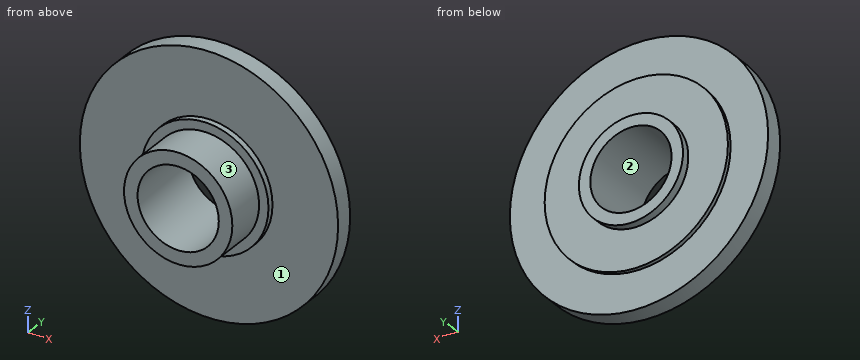
from build123d import *

# Parameters (mm, degrees)
SKETCH3_R          = 19.5
CUT_EXTRUDE1_DEPTH = 50


with BuildPart() as part:
    # Sketch2 → Revolve1 (revolve)
    with BuildSketch(Plane.XY):
        Polygon((0, 0), (26, 0), (26, 20), (30.5, 20), (30.5, 23), (62, 23), (62, 32), (44, 32), (44, 34), (25, 34), (25, 38), (0, 38), align=None)
    revolve(axis=Axis((0, 0, 0), (0, 1, 0)))

    # Sketch3 → Cut-Extrude1 (cut)
    with BuildSketch(Plane(origin=(0, 38, 0), x_dir=(1, 0, 0), z_dir=(0, 1, 0))):
        Circle(SKETCH3_R)
    extrude(amount=-CUT_EXTRUDE1_DEPTH, mode=Mode.SUBTRACT)


solid = part.part
Work out the finished part from the listing and answer in its coordinate system (mm). Face numbers are marked on the shaded views. Give positions to 0.01 mm unless a question says otherwise; leave off trailing zeros. Loops run counter-clockwise (first coordinate to the right, second up) from the corner with the lowest first, then second, coordinate; pieces in that order, holes last. Notation, with made-up numbers: M 36.5,4 L 62.5,4 A31 ccw 62.5,30 Z; hole C -5,44 d3. An arc over 180 degrees is marked long. Use CSV: the item, a comma, the result in double quotes.
1) Consider L1, parallel to Z at x = 0, y = 27; L2, parallel to Y at x = 16.5, z = -39. Determine where each line is inside the solid, lowest interval first.
Answer:
L1,"-62 to -19.5, 19.5 to 62"
L2,"23 to 34"
2) Find section B-B on z = 0. Write down the section's boundary in (x, y), plus the area to 3 significant figures.
Answer:
outline,"M -62,23 L -30.5,23 L -30.5,20 L -26,20 L -26,0 L -19.5,0 L -19.5,38 L -25,38 L -25,34 L -44,34 L -44,32 L -62,32 Z; M 19.5,0 L 26,0 L 26,20 L 30.5,20 L 30.5,23 L 62,23 L 62,32 L 44,32 L 44,34 L 25,34 L 25,38 L 19.5,38 Z"
area,"1,230 mm^2"
3) Determine the mould class of the marked faces 1, 2 and 3 for opening direction X: released by +X, released by -X, zero draft, split by the parting line, or undercut.
Answer:
face 1,"zero draft"
face 2,"undercut"
face 3,"split by the parting line"
4) Find section C-C on x = 34. Write down the section's boundary in (y, z).
Answer:
outline,"M 23,-51.85 L 32,-51.85 L 32,-27.93 L 34,-27.93 L 34,27.93 L 32,27.93 L 32,51.85 L 23,51.85 Z"
5) Given P1, Ø4, axis at x = -5.5, y = 19, coming from the +Z side; P2, Ø3, axis at x = 1.5, y = 29.5, coming from the -Z side; P3, Ø12, axis at y = 12, z = -8, coming from the +X side, each flat-ended and moving along its own axis, determine where each tip first touches the part or whether it passes through.
Answer:
P1,"z = 30.27"
P2,"z = -62"
P3,"x = 25.92"
6) Find section A-A on x = 0. Write down the section's boundary in (y, z), plus the area to 3 significant figures.
Answer:
outline,"M 0,-26 L 20,-26 L 20,-30.5 L 23,-30.5 L 23,-62 L 32,-62 L 32,-44 L 34,-44 L 34,-25 L 38,-25 L 38,-19.5 L 0,-19.5 Z; M 0,19.5 L 38,19.5 L 38,25 L 34,25 L 34,44 L 32,44 L 32,62 L 23,62 L 23,30.5 L 20,30.5 L 20,26 L 0,26 Z"
area,"1,230 mm^2"
7) Find section D-D on y = 10. Write down the section's boundary in (x, z), plus the area to 3 significant figures.
Answer:
outline,"C 0,0 d52; hole C 0,0 d39"
area,"929 mm^2"
